The model under review builds one solid part; all positions refer to its coordinate system, in mm. A direction names the side the tool comes from. Coordinates: 2 decimals unless noted, no trailing zeros. Write each loop counter-clockwise with the first axis right and the second up, starting at its lowest first coordinate (ties: lowest second). Pieces come first, ordered by that corner, then holes. Notation, with made-up numbers: (21.5, 81.25) - (63.5, 81.25) arc R13 cw to (63.5, 89.25) - close; hole circle Ø9 at (-36.5, 15). An arc over 180 degrees is marked (long way). Put each result on its own line as item: value. Start each with the question number.
Item 1: Mouldability with a two-part tool opening along X and no side actions: class faces 1 (the face through (9.61, 2, -25)), 2 (the face through (22, 3, -1.27)), 3 (the face through (-5, 2, 12.36)) as pulls with the +X half, pulls with the -X half, needs draft (parallel to the pull), parting line crosses it, or undercut.
Item 2: Consider section D-D on z = -32.75. Give the boundary of the cut face in (x, y), then the cut area to 3 significant figures.
Item 3: Consider section A-A on x = 7.25. Give the boundary of the cut face in (y, z).
Item 4: To check wall thickness, follow L1, parallel to Z at x = -17.2, y = 1.15; L2, parallel to X at y = 1.65, z = -2; L3, parallel to X at y = 2.05, z = -24.45. State the ranges of each line that lie inside material, in increasing order. Write a range as [from, to].
Item 5: Consider section B-B on z = -16.5. Give the boundary of the cut face in (x, y), then the cut area to 3 significant figures.
Item 6: Consider section C-C on z = 0. Give the boundary of the cut face in (x, y), then the cut area to 3 significant figures.
Item 7: For pin 1 (3 mm diameter, centred on x = -18, y = 1, fed in from -Z); pin 2 (15.5 mm diameter, centred on x = 23.5, z = -5, fed in from +Y); pin 3 (3 mm diameter, centred on y = 1, z = -14.5, fed in from -X), all flat-tipped, find the tip position at first contact; note any pin that passes through.
Item 8: Machinability: for faces 4 (the face through (11.11, 2.03, -41.43)), 5 (the face through (22, 2, -20.27)), 6 (the face through (22.181, 3.282, -38.245)), which of the approach directions +Z, -Z, +X, -X, +Y, -Y give a long, thin tool a straight path to every point of the face, cutting with its end or side? Answer none if there is none.
```python
from build123d import *

# Parameters (mm, degrees)
EXTRUDE_1_DEPTH          = 4
CUT_EXTRUDE_1_DEPTH      = 38.905694823
CUT_EXTRUDE_1_DEPTH_BACK = 38.905694823
SKETCH_2_R               = 1
SKETCH_3_W               = 14
SKETCH_3_H               = 20.72
CUT_EXTRUDE_3_DEPTH      = 3
SKETCH_5_W               = 5
SKETCH_5_H               = 20.72
CUT_EXTRUDE_4_DEPTH      = 4
SKETCH_6_R               = 9
EXTRUDE_2_DEPTH          = 1.5
SKETCH_10_R              = 5.5
CUT_EXTRUDE_6_DEPTH      = 3.5
SKETCH_12_W              = 24.72
SKETCH_12_H              = 4
EXTRUDE_3_DEPTH          = 24.72
SKETCH_14_W              = 24.72
SKETCH_14_H              = 4
EXTRUDE_4_DEPTH          = 30.5
SKETCH_15_R              = 1
SKETCH_15_R_2            = 5.5
CUT_EXTRUDE_7_DEPTH      = 4
EXTRUDE_START            = 1.5
SKETCH_16_R              = 9
SKETCH_16_R_2            = 5.5
EXTRUDE_5_DEPTH          = 1.5
SKETCH_17_W              = 20.72
SKETCH_17_H              = 19
CUT_EXTRUDE_8_DEPTH      = 4
SKETCH_19_W              = 20.72
SKETCH_19_H              = 14
EXTRUDE_6_DEPTH          = 1
EXTRUDE_START_2          = -1
SKETCH_20_R              = 5.5
EXTRUDE_7_DEPTH          = 1
FILLET_1_R               = 5
FILLET_2_R               = 5
FILLET_6_R               = 10


with BuildPart() as part:
    # 草图1 → 凸台-拉伸1 (new body)
    with BuildSketch(Plane(origin=(0, 0, 0), x_dir=(1, 0, 0), z_dir=(0, 1, 0))):
        with BuildLine():
            Line((6.61, -12.36), (9.61, -12.36))
            Line((9.61, -12.36), (9.61, -9.36))
            Line((9.61, -9.36), (9.61, 9.36))
            Line((9.61, 9.36), (9.61, 12.36))
            Line((9.61, 12.36), (6.61, 12.36))
            Line((6.61, 12.36), (-32.61, 12.36))
            ThreePointArc((-32.61, 12.36), (-34.731320344, 11.481320344), (-35.61, 9.36))
            Line((-35.61, 9.36), (-35.61, -9.36))
            ThreePointArc((-35.61, -9.36), (-34.731320344, -11.481320344), (-32.61, -12.36))
            Line((-32.61, -12.36), (6.61, -12.36))
        make_face()
    extrude(amount=EXTRUDE_1_DEPTH)

    # 草图2 → 切除-拉伸1 (cut, two sides: drawn at the far end of the back side and taken through both)
    with BuildSketch(Plane(origin=(0, 0, 0), x_dir=(1, 0, 0), z_dir=(0, 1, 0)).offset(-CUT_EXTRUDE_1_DEPTH_BACK)):
        with Locations(Location((7.25, -10.25, 0), (0, 0, 270))):
            Circle(SKETCH_2_R)
        with Locations(Location((7.25, 10.25, 0), (0, 0, 270))):
            Circle(SKETCH_2_R)
        with Locations(Location((-17.2, -10.25, 0), (0, 0, 270))):
            Circle(SKETCH_2_R)
        with Locations(Location((-17.2, 10.25, 0), (0, 0, 270))):
            Circle(SKETCH_2_R)
    extrude(amount=CUT_EXTRUDE_1_DEPTH + CUT_EXTRUDE_1_DEPTH_BACK, mode=Mode.SUBTRACT)

    # 草图3 → 切除-拉伸3 (cut)
    with BuildSketch(Plane(origin=(0, 4, 0), x_dir=(1, 0, 0), z_dir=(0, 1, 0))):
        with Locations((-1.39, 0)):
            Rectangle(SKETCH_3_W, SKETCH_3_H)
    extrude(amount=-CUT_EXTRUDE_3_DEPTH, mode=Mode.SUBTRACT)

    # 草图5 → 切除-拉伸4 (cut)
    with BuildSketch(Plane(origin=(0, 4, 0), x_dir=(1, 0, 0), z_dir=(0, 1, 0))):
        with Locations((-10.89, 0)):
            Rectangle(SKETCH_5_W, SKETCH_5_H)
    extrude(amount=-CUT_EXTRUDE_4_DEPTH, mode=Mode.SUBTRACT)

    # 草图6 → 凸台-拉伸2 (add)
    with BuildSketch(Plane(origin=(0, 4, 0), x_dir=(1, 0, 0), z_dir=(0, 1, 0))):
        with Locations(Location((-25.5, 0, 0), (0, 0, 270))):
            Circle(SKETCH_6_R)
    extrude(amount=EXTRUDE_2_DEPTH)

    # 草图10 → 切除-拉伸6 (cut)
    with BuildSketch(Plane(origin=(0, 5.5, 0), x_dir=(1, 0, 0), z_dir=(0, 1, 0))):
        with Locations(Location((-25.62236192, 0, 0), (0, 0, 270))):
            Circle(SKETCH_10_R)
    extrude(amount=-CUT_EXTRUDE_6_DEPTH, mode=Mode.SUBTRACT)

    # 草图12 → 凸台-拉伸3 (add)
    with BuildSketch(Plane(origin=(9.61, 0, 0), x_dir=(0, 0, -1), z_dir=(1, 0, 0))):
        with Locations((0, 2)):
            Rectangle(SKETCH_12_W, SKETCH_12_H)
    extrude(amount=EXTRUDE_3_DEPTH)

    # 草图14 → 凸台-拉伸4 (add)
    with BuildSketch(Plane(origin=(0, 0, -12.36), x_dir=(-1, 0, 0), z_dir=(0, 0, -1))):
        with Locations((-21.97, 2)):
            Rectangle(SKETCH_14_W, SKETCH_14_H)
    extrude(amount=EXTRUDE_4_DEPTH)

    # 草图15 → 切除-拉伸7 (cut)
    with BuildSketch(Plane(origin=(0, 4, 0), x_dir=(1, 0, 0), z_dir=(0, 1, 0))):
        with Locations(Location((11.72, 24.45, 0), (0, 0, 270))):
            Circle(SKETCH_15_R)
        with Locations(Location((32.22, 24.45, 0), (0, 0, 270))):
            Circle(SKETCH_15_R)
        with Locations(Location((11.72, 0, 0), (0, 0, 270))):
            Circle(SKETCH_15_R)
        with Locations(Location((32.22, 0, 0), (0, 0, 270))):
            Circle(SKETCH_15_R)
        with Locations(Location((21.938853273, 32.75, 0), (0, 0, 270))):
            Circle(SKETCH_15_R_2)
    extrude(amount=-CUT_EXTRUDE_7_DEPTH, mode=Mode.SUBTRACT)

    # 草图16 → 凸台-拉伸5 (add)
    with BuildSketch(Plane(origin=(0, 4, 0), x_dir=(1, 0, 0), z_dir=(0, 1, 0)).offset(EXTRUDE_START)):
        with Locations(Location((21.938853273, 32.75, 0), (0, 0, 270))):
            Circle(SKETCH_16_R)
        with Locations(Location((21.938853273, 32.75, 0), (0, 0, 270))):
            Circle(SKETCH_16_R_2, mode=Mode.SUBTRACT)
    extrude(amount=-EXTRUDE_5_DEPTH)

    # 草图17 → 切除-拉伸8 (cut)
    with BuildSketch(Plane(origin=(0, 4, 0), x_dir=(1, 0, 0), z_dir=(0, 1, 0))):
        with Locations((21.97, 10.77)):
            Rectangle(SKETCH_17_W, SKETCH_17_H)
    extrude(amount=-CUT_EXTRUDE_8_DEPTH, mode=Mode.SUBTRACT)

    # 草图19 → 凸台-拉伸6 (add)
    with BuildSketch(Plane.XZ):
        with Locations((21.97, -8.27)):
            Rectangle(SKETCH_19_W, SKETCH_19_H)
    extrude(amount=-EXTRUDE_6_DEPTH)

    # 草图20 → 凸台-拉伸7 (add)
    with BuildSketch(Plane.XZ.offset(EXTRUDE_START_2)):
        with Locations(Location((21.938853273, -32.75, 0), (0, 0, 90))):
            Circle(SKETCH_20_R)
    extrude(amount=EXTRUDE_7_DEPTH)

    # 圆角1
    fillet_1_edges = [part.edges().sort_by_distance(p)[0] for p in [
        (34.33, 2, -42.86),
    ]]
    fillet(fillet_1_edges, radius=FILLET_1_R)

    # 圆角2
    fillet_2_edges = [part.edges().sort_by_distance(p)[0] for p in [
        (9.61, 2, -42.86),
    ]]
    fillet(fillet_2_edges, radius=FILLET_2_R)

    # 圆角6
    fillet_6_edges = [part.edges().sort_by_distance(p)[0] for p in [
        (34.33, 2, 12.36),
    ]]
    fillet(fillet_6_edges, radius=FILLET_6_R)


solid = part.part
```
Report:
1. face 1: pulls with the -X half
1. face 2: undercut
1. face 3: needs draft
2. outline: (9.61, 0) - (34.33, 0) - (34.33, 4) - (30.94, 4) - (30.94, 5.5) - (27.44, 5.5) - (27.44, 1) - (16.44, 1) - (16.44, 5.5) - (12.94, 5.5) - (12.94, 4) - (9.61, 4) - close
2. area: 76.4 mm²
3. outline: (0, -12.36) - (4, -12.36) - (4, -11.25) - (0, -11.25) - close; (0, -9.25) - (4, -9.25) - (4, 9.25) - (0, 9.25) - close; (0, 11.25) - (4, 11.25) - (4, 12.36) - (0, 12.36) - close
4. L1: [-12.36, -11.25], [-9.25, 9.25], [11.25, 12.36]
4. L2: [-35.61, -13.39], [5.61, 11.61], [32.33, 34.33]
4. L3: [9.61, 10.72], [12.72, 31.22], [33.22, 34.33]
5. outline: (9.61, 0) - (11.61, 0) - (11.61, 4) - (9.61, 4) - close; (32.33, 0) - (34.33, 0) - (34.33, 4) - (32.33, 4) - close
5. area: 16.0 mm²
6. outline: (-35.61, 0) - (-13.39, 0) - (-13.39, 4) - (-16.5, 4) - (-16.5, 5.5) - (-20.12, 5.5) - (-20.12, 2) - (-31.12, 2) - (-31.12, 5.5) - (-34.5, 5.5) - (-34.5, 4) - (-35.61, 4) - close; (-8.39, 0) - (10.72, 0) - (10.72, 4) - (5.61, 4) - (5.61, 1) - (-8.39, 1) - close; (12.72, 0) - (31.22, 0) - (31.22, 4) - (12.72, 4) - close; (33.22, 0) - (34.33, 0) - (34.33, 4) - (33.22, 4) - close
6. area: 190 mm²
7. pin 1: z = -12.36
7. pin 2: y = 4
7. pin 3: x = 9.61
8. face 4: -Z, -X, +Y, -Y
8. face 5: +Y, -Y
8. face 6: +Y
